Work out the finished part from the listing and answer in its coordinate system (mm). Face numbers are marked on the shaded views. A direction names the side the tool comes from. Give positions to 0.01 mm unless a question says otherwise; leave off trailing zeros. Loops run counter-clockwise (first coordinate to the right, second up) from the corner with the lowest first, then second, coordinate; pieces in that order, holes last.
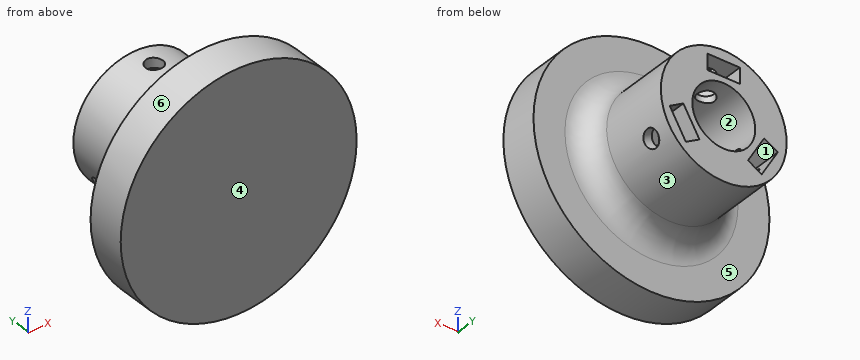
from build123d import *

# Parameters (mm, degrees)
SKETCH4_W          = 1.1
SKETCH4_H          = 20.490381057
CUT_EXTRUDE1_START = -1.25
CUT_EXTRUDE1_DEPTH = 2
CIRPATTERN1_COUNT  = 3
FILLET1_R          = 3


with BuildPart() as part:
    # Sketch1 → Revolve1 (revolve)
    with BuildSketch(Plane.XY, mode=Mode.PRIVATE) as revolve1_sk:
        Polygon((0, 0), (15, 0), (15, 5), (8, 5), (8, 17), (4, 17), (4, 5), (0, 5), align=None)
    revolve(revolve1_sk.sketch.rotate(Axis((0, 0, 0), (0, 1, 0)), 90), axis=Axis((0, 0, 0), (0, 1, 0)))

    # Sketch4 → M2 Clearance Hole1 (revolve, cut)
    with BuildSketch(Plane(origin=(0, 14, 0), x_dir=(0, 1, 0), z_dir=(1, 0, 0))):
        with Locations((0.55, 10.245190529)):
            Rectangle(SKETCH4_W, SKETCH4_H)
    m2_clearance_hole1 = revolve(axis=Axis((0, 14, -6.35), (0, 0, 1)), mode=Mode.SUBTRACT)

    # Sketch5 → Cut-Extrude1 (cut)
    with BuildSketch(Plane.XY.offset(8).offset(CUT_EXTRUDE1_START)):
        Polygon((2.05, 17), (2.05, 15.183568052), (0, 16.367136104), (-2.05, 15.183568052), (-2.05, 17), align=None)
        Polygon((0, 11.632863896), (2.05, 12.816431948), (2.05, 15.183568052), (0, 16.367136104), (-2.05, 15.183568052), (-2.05, 12.816431948), align=None)
    cut_extrude1 = extrude(amount=-CUT_EXTRUDE1_DEPTH, mode=Mode.SUBTRACT)

    # CirPattern1: M2 Clearance Hole1, Cut-Extrude1 ×3 about axis
    cirpattern1_axis = Axis((0, 0, 0), (0, 1, 0))
    add([m2_clearance_hole1.rotate(cirpattern1_axis, i * 360 / CIRPATTERN1_COUNT) for i in range(1, CIRPATTERN1_COUNT)], mode=Mode.SUBTRACT)
    add([cut_extrude1.rotate(cirpattern1_axis, i * 360 / CIRPATTERN1_COUNT) for i in range(1, CIRPATTERN1_COUNT)], mode=Mode.SUBTRACT)

    # Fillet1
    fillet1_edges = [part.edges().sort_by_distance(p)[0] for p in [
        (0, 5, 8),
    ]]
    fillet(fillet1_edges, radius=FILLET1_R)


solid = part.part
Item 1: Flat-ended cylindrical pins translate along their axes: pin 1 Ø2 at (y, z) = (15.5, 5.5) entering from -X; pin 2 Ø2.5 at (x, y) = (0, 14) entering from +Z; pin 3 Ø0.6 at (y, z) = (15.5, 6) entering from +X; pin 4 Ø3 at (y, z) = (14, 11) entering from +X. Find the tip coordinate at first contact, or state that the pin passes through.
Item 2: Find section C-C, the plane y = 10. Write down the section's boundary in (x, z), plus the area to 3 significant figures.
Item 3: Consider line 1 (Y direction, x = 0, z = 7.7); line 2 (X direction, y = 12.75, z = -0.25); line 3 (X direction, y = 14.75, z = 5) (3 decimals). Determine where each line is inside the solid, lowest interval first.
Item 4: Find section D-D, the plane y = 14. Give the number of separate pieces and of enclosed holes in the cut face, plus the area to 3 significant figures.
Item 5: Determine the mould class of the marked faces 1, 2, 3 and 4 for opening direction X: released by +X, released by -X, zero draft, split by the parting line, or undercut.
Item 6: Find section A-A, the plane y = 16. Write down the section's boundary in (x, z).
Item 7: For the marked faces 5 and 6, determine the directions among +Z, -Z, +X, -X, +Y, -Y from which every point of the face is accessible in a straight line to the end or side of a thin tool.
Item 8: Find section B-B, the plane z = 0. Write down the section's boundary in (x, y).
Ans:
1. pin 1: stops at x = -6.61
1. pin 2: stops at z = 8
1. pin 3: stops at x = 5.61
1. pin 4: passes through
2. outline: circle Ø16 at (0, 0); hole circle Ø8 at (0, 0)
2. area: 151 mm2
3. line 1: y = 0 to 12.9, 15.1 to 17
3. line 2: x = -8 to -3.99, 3.99 to 8
3. line 3: x = -6.245 to -2.05, 2.05 to 6.245
4. separate pieces: 3
4. enclosed holes: 0
4. area: 113 mm2
5. face 1: undercut
5. face 2: undercut
5. face 3: split by the parting line
5. face 4: zero draft
6. outline: circle Ø16 at (0, 0); hole (-6.87, -1.6) - (-4.82, -5.15) - (-3.09, -4.15) - (-5.14, -0.6) - close; hole circle Ø8 at (0, 0); hole (-2.05, 4.75) - (2.05, 4.75) - (2.05, 6.75) - (-2.05, 6.75) - close; hole (3.09, -4.15) - (4.82, -5.15) - (6.87, -1.6) - (5.14, -0.6) - close
7. face 5: +Y
7. face 6: +Y, -Y
8. outline: (-15, 0) - (15, 0) - (15, 5) - (11, 5) arc R3 cw to (8, 8) - (8, 17) - (4, 17) - (4, 5) - (-4, 5) - (-4, 17) - (-8, 17) - (-8, 8) arc R3 cw to (-11, 5) - (-15, 5) - close
